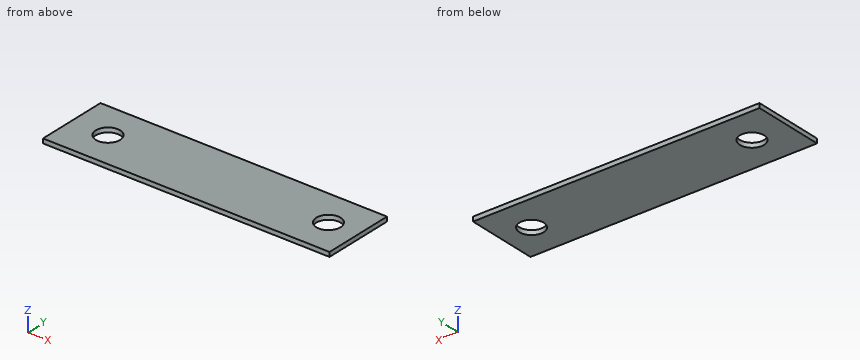
```python
from build123d import *

# Parameters (mm, degrees)
F1_DEPTH = 2.38125


# Not quite as in the source:
# - a feature names something its author has since deleted; it is built from what else it names


with BuildPart() as f1:
    # F0 (on Top) → F1 (new body)
    with BuildSketch(Plane.XY):
        with BuildLine():
            Line((-9.4234, 38.1), (0, 38.1))
            Line((0, 38.1), (0, 57.15))
            Line((0, 57.15), (-152.4, 57.15))
            Line((-152.4, 57.15), (-152.4, 38.1))
            Line((-152.4, 38.1), (-139.5476, 38.1))
            ThreePointArc((-139.5476, 38.1), (-133.096, 44.5516), (-126.6444, 38.1))
            Line((-126.6444, 38.1), (-22.3266, 38.1))
            ThreePointArc((-22.3266, 38.1), (-15.875, 44.5516), (-9.4234, 38.1))
        make_face()
        with BuildLine():
            Line((-152.4, 19.05), (0, 19.05))
            Line((0, 19.05), (0, 38.1))
            Line((0, 38.1), (-9.4234, 38.1))
            ThreePointArc((-9.4234, 38.1), (-15.875, 31.6484), (-22.3266, 38.1))
            Line((-22.3266, 38.1), (-126.6444, 38.1))
            ThreePointArc((-126.6444, 38.1), (-133.096, 31.6484), (-139.5476, 38.1))
            Line((-139.5476, 38.1), (-152.4, 38.1))
            Line((-152.4, 38.1), (-152.4, 19.05))
        make_face()
    extrude(amount=F1_DEPTH)


solid = f1.part
```
Geometry check sheet. Reference: the model listing, model coordinates, mm. Give positions to 0.01 mm unless a question says otherwise; leave off trailing zeros. Write each loop counter-clockwise with the first axis right and the second up, starting at its lowest first coordinate (ties: lowest second). Pieces come first, ordered by that corner, then holes.
1) Section check B-B, the plane z = 1.3. Record the boundary of the cut face in (x, y) (3 decimals), and give its area (3 significant figures).
2) Section check A-A, the plane y = 38.1. Record the boundary of the cut face in (x, z).
3) Material ranges on L1, parallel to X at y = 38.1, z = 1.7; L2, parallel to X at y = 37.5, z = 0.7; L3, parallel to Y at x = -130.5, z = 0.45, recorded low to high.
Computed:
1. outline: (-152.4, 19.05) - (0, 19.05) - (0, 57.15) - (-152.4, 57.15) - close; hole circle Ø12.903 at (-133.096, 38.1); hole circle Ø12.903 at (-15.875, 38.1)
1. area: 5,540 mm2
2. outline: (-152.4, 0) - (-139.55, 0) - (-139.55, 2.38) - (-152.4, 2.38) - close; (-126.64, 0) - (-22.33, 0) - (-22.33, 2.38) - (-126.64, 2.38) - close; (-9.42, 0) - (0, 0) - (0, 2.38) - (-9.42, 2.38) - close
3. L1: x = -152.4 to -139.55, -126.64 to -22.33, -9.42 to 0
3. L2: x = -152.4 to -139.52, -126.67 to -22.3, -9.45 to 0
3. L3: y = 19.05 to 32.19, 44.01 to 57.15
